```python
from build123d import *

# Parameters (mm, degrees)
SKETCH3_W           = 14
SKETCH3_H           = 6.5
BOSS_EXTRUDE2_DEPTH = 8
CUT_EXTRUDE1_START  = 2
CUT_EXTRUDE1_DEPTH  = 6
LPATTERN2_COUNT     = 7
LPATTERN2_PITCH     = 2
SKETCH4_W           = 14
SKETCH4_H           = 7
SKETCH4_R           = 1.6
BOSS_EXTRUDE3_DEPTH = 2
SKETCH5_W           = 5
SKETCH5_H           = 8
BOSS_EXTRUDE4_DEPTH = 7.5
SKETCH6_R           = 1.6
CUT_EXTRUDE2_DEPTH  = 7.5


with BuildPart() as part:
    # Sketch3 → Boss-Extrude2 (new body)
    with BuildSketch(Plane.XY):
        with Locations((7, 1.25)):
            Rectangle(SKETCH3_W, SKETCH3_H)
    extrude(amount=BOSS_EXTRUDE2_DEPTH)

    # Sketch1 → Cut-Extrude1 (cut)
    with BuildSketch(Plane.XY.offset(CUT_EXTRUDE1_START)):
        with BuildLine():
            Line((0.740175425, 0.63), (1.259824575, 0.63))
            ThreePointArc((1.259824575, 0.63), (1.358731646, 0.667228588), (1.408543109, 0.760434783))
            ThreePointArc((1.408543109, 0.760434783), (1.442388286, 0.918062154), (1.501123596, 1.068202247))
            ThreePointArc((1.501123596, 1.068202247), (1.705850588, 1.295639059), (2, 1.38))
            Line((2, 1.38), (2, 0))
            Line((2, 0), (0, 0))
            Line((0, 0), (0, 1.38))
            ThreePointArc((0, 1.38), (0.294149412, 1.295639059), (0.498876404, 1.068202247))
            ThreePointArc((0.498876404, 1.068202247), (0.557611714, 0.918062154), (0.591456891, 0.760434783))
            ThreePointArc((0.591456891, 0.760434783), (0.641268354, 0.667228588), (0.740175425, 0.63))
        make_face()
    cut_extrude1 = extrude(amount=CUT_EXTRUDE1_DEPTH, mode=Mode.SUBTRACT)

    # LPattern2: Cut-Extrude1 ×7
    with Locations(*[(i * LPATTERN2_PITCH, 0, 0) for i in range(1, LPATTERN2_COUNT)]):
        add(cut_extrude1, mode=Mode.SUBTRACT)

    # Sketch4 → Boss-Extrude3 (add)
    with BuildSketch(Plane(origin=(0, 4.5, 0), x_dir=(-1, 0, 0), z_dir=(0, 1, 0))):
        with Locations((-7, -3.5)):
            Rectangle(SKETCH4_W, SKETCH4_H)
        with Locations((-10.5, -3.5)):
            Circle(SKETCH4_R, mode=Mode.SUBTRACT)
        with Locations((-3.5, -3.5)):
            Circle(SKETCH4_R, mode=Mode.SUBTRACT)
    extrude(amount=-BOSS_EXTRUDE3_DEPTH)

    # Sketch5 → Boss-Extrude4 (add)
    with BuildSketch(Plane.XZ.offset(2)):
        with Locations((11.5, 4)):
            Rectangle(SKETCH5_W, SKETCH5_H)
    extrude(amount=BOSS_EXTRUDE4_DEPTH)

    # Sketch6 → Cut-Extrude2 (cut)
    with BuildSketch(Plane.ZY.offset(-9)):
        with Locations((4, -5.75)):
            Circle(SKETCH6_R)
    extrude(amount=-CUT_EXTRUDE2_DEPTH, mode=Mode.SUBTRACT)


solid = part.part
```
Design review of the part built by this model. Coordinates are the model's own, in mm. A direction names the side the tool comes from. Round coordinates to 2 decimals unless told otherwise and drop trailing zeros. Order: outer loops, then holes, each group sorted by start corner. A loop starts at its lowest first (then second) coordinate and runs counter-clockwise, first axis right, second up. Notation, with made-up numbers: (2.5, -1.5) - (52.5, -1.5) arc R17 ccw to (52.5, 12.5) - close; hole circle Ø8 at (15, 77). An arc over 180 degrees is marked (long way). Return JSON: item names as keys, results as strings.
Q1. For pin 1 Ø2 at (x, z) = (4, -2.5) entering from -Y; pin 2 Ø4 at (y, z) = (-5.75, 4) entering from -X; pin 3 Ø0.6 at (x, z) = (1, 4) entering from -Y, all flat-tipped, find the tip position at first contact; note any pin that passes through.
Computed values:
{"pin 1": "stops at y = 2.5", "pin 2": "stops at x = 9", "pin 3": "stops at y = -2"}
Q2. Machinability: for faces 1 (the flat face through (7, 0, 5)), 2 (the flat face through (7, 2.5, -3)), 3 (the flat face through (9, -4, 4)), which of the approach directions +Z, -Z, +X, -X, +Y, -Y give a long, thin tool a straight path to every point of the face, cutting with its end or side? Answer none if there is none.
Computed values:
{"face 1": "+Z, +X, -X", "face 2": "-Z, +X, -X, -Y", "face 3": "+Z, -Z, -X, -Y"}
Q3. Consider section B-B on x = 11.75. Write out the cut boundary in (y, z).
Computed values:
{"outline": "(-9.5, 0) - (2.5, 0) - (2.5, -2.5) - (4.5, -2.5) - (4.5, 8) - (1.32, 8) - (1.32, 2) - (0, 2) - (0, 8) - (-9.5, 8) - close; (2.5, -7) - (4.5, -7) - (4.5, -4.5) - (2.5, -4.5) - close; hole circle Ø3.2 at (-5.75, 4)"}
Q4. Consider section C-C on y = -5.75. Write out the cut boundary in (x, z).
Computed values:
{"outline": "(9, 0) - (14, 0) - (14, 2.4) - (9, 2.4) - close; (9, 5.6) - (14, 5.6) - (14, 8) - (9, 8) - close"}
Q5. The part is to be moulded in two halves that separate along Y. For faces 4 (the flat face through (8, -1, 0)), 5 (the flat face through (7.1, 0.4, 2)), 6 (the flat face through (4, -2, 4)), say which applies: pulls with the +Y half, pulls with the -Y half, needs draft (parallel to the pull), parting line crosses it, or undercut.
Computed values:
{"face 4": "needs draft", "face 5": "undercut", "face 6": "pulls with the -Y half"}
Q6. Consider section D-D on x = 3. Write out the cut boundary in (y, z).
Computed values:
{"outline": "(-2, 0) - (2.5, 0) - (2.5, -1.98) - (4.5, -1.98) - (4.5, 8) - (0.63, 8) - (0.63, 2) - (0, 2) - (0, 8) - (-2, 8) - close; (2.5, -7) - (4.5, -7) - (4.5, -5.02) - (2.5, -5.02) - close"}
Q7. Wall thickness on L1, parallel to Y at x = 11.3, z = 4; L2, parallel to Z at x = 3.5, y = 4; L3, parallel to Y at x = 2, z = 7.25: over which ranges is each line inside the solid? List them lowest first. Write a range as [from, to].
Computed values:
{"L1": "y = [-9.5, -7.35], [-4.15, 0], [0.64, 4.5]", "L2": "z = [-7, -5.1], [-1.9, 8]", "L3": "y = [-2, 0], [1.38, 4.5]"}
Q8. Consider section A-A on z = -3.5. Write out the cut boundary in (x, y), plus the area to 3 significant figures.
Computed values:
{"outline": "(0, 2.5) - (1.9, 2.5) - (1.9, 4.5) - (0, 4.5) - close; (5.1, 2.5) - (8.9, 2.5) - (8.9, 4.5) - (5.1, 4.5) - close; (12.1, 2.5) - (14, 2.5) - (14, 4.5) - (12.1, 4.5) - close", "area": "15.2 mm2"}
